from build123d import *

# Parameters (mm, degrees)
SKETCH1_R           = 7
SKETCH1_R_2         = 5
BOSS_EXTRUDE1_DEPTH = 3
SKETCH1_3_R         = 5
BOSS_EXTRUDE2_DEPTH = 8
BOSS_EXTRUDE3_START = -8
BOSS_EXTRUDE3_DEPTH = 10


with BuildPart() as part:
    # Sketch1 → Boss-Extrude1 (new body)
    # profile 1 of 4: a face of its own
    with BuildSketch(Plane(origin=(0, 0, 0), x_dir=(1, 0, 0), z_dir=(0, 1, 0))):
        with Locations(Location((0, 0, 0), (0, 0, 270))):
            Circle(SKETCH1_R)
        Circle(SKETCH1_R_2, mode=Mode.SUBTRACT)
    # profile 2 of 4: a face of its own
    with BuildSketch(Plane(origin=(0, 0, 0), x_dir=(1, 0, 0), z_dir=(0, 1, 0))):
        Circle(SKETCH1_R_2)
        with BuildLine():
            ThreePointArc((-1.85, -1.966596044), (0, -2.7), (1.85, -1.966596044))
            Line((1.85, -1.966596044), (1.85, 1.966596044))
            ThreePointArc((1.85, 1.966596044), (0, 2.7), (-1.85, 1.966596044))
            Line((-1.85, 1.966596044), (-1.85, -1.966596044))
        make_face(mode=Mode.SUBTRACT)
    # profile 3 of 4: a face of its own
    with BuildSketch(Plane(origin=(0, 0, 0), x_dir=(1, 0, 0), z_dir=(0, 1, 0))):
        with BuildLine():
            Line((1.85, -1.966596044), (1.85, 1.966596044))
            ThreePointArc((1.85, 1.966596044), (0.995035346, 2.509961087), (0, 2.7))
            Line((0, 2.7), (0, -2.7))
            ThreePointArc((0, -2.7), (0.995035346, -2.509961087), (1.85, -1.966596044))
        make_face()
    # profile 4 of 4: a face of its own
    with BuildSketch(Plane(origin=(0, 0, 0), x_dir=(1, 0, 0), z_dir=(0, 1, 0))):
        with BuildLine():
            Line((0, -2.7), (0, 2.7))
            ThreePointArc((0, 2.7), (-0.995035346, 2.509961087), (-1.85, 1.966596044))
            Line((-1.85, 1.966596044), (-1.85, -1.966596044))
            ThreePointArc((-1.85, -1.966596044), (-0.995035346, -2.509961087), (0, -2.7))
        make_face()
    extrude(amount=BOSS_EXTRUDE1_DEPTH)

    # Sketch1<3> → Boss-Extrude2 (add)
    with BuildSketch(Plane(origin=(0, 0, 0), x_dir=(1, 0, 0), z_dir=(0, 1, 0))):
        with Locations(Location((0, 0, 0), (0, 0, 270))):
            Circle(SKETCH1_3_R)
    extrude(amount=-BOSS_EXTRUDE2_DEPTH)

    # Sketch1<5> → Boss-Extrude3 (add)
    with BuildSketch(Plane(origin=(0, 0, 0), x_dir=(1, 0, 0), z_dir=(0, 1, 0)).offset(BOSS_EXTRUDE3_START)):
        with BuildLine():
            Line((0, -2.7), (0, 2.7))
            ThreePointArc((0, 2.7), (-0.995035346, 2.509961087), (-1.85, 1.966596044))
            Line((-1.85, 1.966596044), (-1.85, -1.966596044))
            ThreePointArc((-1.85, -1.966596044), (-0.995035346, -2.509961087), (0, -2.7))
        make_face()
        with BuildLine():
            Line((1.85, -1.966596044), (1.85, 1.966596044))
            ThreePointArc((1.85, 1.966596044), (0.995035346, 2.509961087), (0, 2.7))
            Line((0, 2.7), (0, -2.7))
            ThreePointArc((0, -2.7), (0.995035346, -2.509961087), (1.85, -1.966596044))
        make_face()
    extrude(amount=-BOSS_EXTRUDE3_DEPTH)


solid = part.part
Read the model definition and answer for the solid it produces. Units are mm, in the model's axes. A direction names the side the tool comes from. Coordinates: 2 decimals unless noted, no trailing zeros. Order: outer loops, then holes, each group sorted by start corner. A loop starts at its lowest first (then second) coordinate and runs counter-clockwise, first axis right, second up. Notation, with made-up numbers: (77.25, -4.5) - (104.25, -4.5) arc R21 ccw to (104.25, 3.5) - close; hole circle Ø5 at (62, -35). An arc over 180 degrees is marked (long way). Use one line per item in the form item = value.
(1) Given pin 1 Ø4.5 at (y, z) = (-14.5, -0.5) entering from +X; pin 2 Ø4.5 at (y, z) = (-11.5, 0) entering from -X; pin 3 Ø2 at (y, z) = (-1.5, -2) entering from -X, each flat-ended and moving along its own axis, determine where each tip first touches the part or whether it passes through.
Computed values:
pin_1 = 1.85
pin_2 = -1.85
pin_3 = -4.9
(2) Section D-D, the plane z = 3.5 is taken. Give the vertices of the cut face in (x, y), then the cut area to 3 significant figures.
Computed values:
outline = (-6.06, 0) - (-3.57, 0) - (-3.57, -8) - (3.57, -8) - (3.57, 0) - (6.06, 0) - (6.06, 3) - (-6.06, 3) - close
area = 93.5 mm²
(3) Which of the six approach directions +Z, -Z, +X, -X, +Y, -Y give full straight-line access (tool end or side, diameter ignored) to faces 1 (the face through (1.85, -13, 0)), 2 (the face through (-2, 0, -5)), 3 (the face through (0, -18, 0)), 4 (the face through (-1.85, -13, 0))?
Computed values:
face_1 = +Z, -Z, +X, -Y
face_2 = -Y
face_3 = +Z, -Z, +X, -X, -Y
face_4 = +Z, -Z, -X, -Y
(4) Section B-B, the plane y = -8.75 is taken. Give the vertices of the cut face in (x, z), then the cut area to 3 significant figures.
Computed values:
outline = (-1.85, -1.97) arc R2.7 ccw to (1.85, -1.97) - (1.85, 1.97) arc R2.7 ccw to (-1.85, 1.97) - close
area = 18.3 mm²
(5) Section C-C, the plane x = -4.25 is taken. Give the vertices of the cut face in (y, z).
Computed values:
outline = (-8, -2.63) - (0, -2.63) - (0, -5.56) - (3, -5.56) - (3, 5.56) - (0, 5.56) - (0, 2.63) - (-8, 2.63) - close
(6) Straight lines are drawn through the part: L1, parallel to Y at x = -4, z = 0.5; L2, parallel to Y at x = -4.25, z = -3.5; L3, parallel to X at y = -8.5, z = 1.5. For each, find the intervals that lie inside material, in ascending order.
Computed values:
L1 = -8 to 3
L2 = 0 to 3
L3 = -1.85 to 1.85
(7) Section A-A, the plane z = 0 is taken. Give the vertices of the cut face in (x, y), then the cut area to 3 significant figures.
Computed values:
outline = (-7, 0) - (-5, 0) - (-5, -8) - (-1.85, -8) - (-1.85, -18) - (1.85, -18) - (1.85, -8) - (5, -8) - (5, 0) - (7, 0) - (7, 3) - (-7, 3) - close
area = 159 mm²
